```python
from build123d import *

# Parameters (mm, degrees)
F0_R     = 36.4281701053
F0_R_2   = 16.7456603081
F1_DEPTH = 984.504
F2_DEPTH = 127


# Not quite as in the source:
# - a feature of the source that left no trace in its solid (it failed there, or was rolled back) is left out
# - the program builds the solid bodies; features that only make, move or delete a surface that nothing else refers to are left out


with BuildPart() as f1:
    # F0 (on Front) → F1 (new body)
    with BuildSketch(Plane.XZ):
        Circle(F0_R)
        Circle(F0_R_2, mode=Mode.SUBTRACT)
    extrude(amount=F1_DEPTH)

    # F0 (on Front) → F2 (join)
    with BuildSketch(Plane.XZ):
        Polygon((0.0695483181, -76.0122935755), (65.8633513954, -37.9459161775), (65.7938030773, 38.0663773981), (-0.0695483181, 76.0122935755), (-65.8633513954, 37.9459161775), (-65.7938030773, -38.0663773981), align=None)
        Circle(F0_R, mode=Mode.SUBTRACT)
    extrude(amount=F2_DEPTH)


solid = f1.part
```
Work out the finished part from the listing and answer in its coordinate system (mm). A direction names the side the tool comes from. Give positions to 0.01 mm unless a question says otherwise; leave off trailing zeros. Order: outer loops, then holes, each group sorted by start corner. A loop starts at its lowest first (then second) coordinate and runs counter-clockwise, first axis right, second up. Notation, with made-up numbers: (87.25, 19) - (120.25, 19) arc R22 ccw to (120.25, 45) - close; hole circle Ø9 at (26.5, -20). An arc over 180 degrees is marked (long way). One line per item, written item: value. Start each with the question number.
1. For a pull along Z with two mould halves and no side action, classify faces 1 (the face through (-16, -127, 35)), 2 (the face through (-33.323, -62.611, -56.774)), 3 (the face through (-32.506, -62.611, 57.246)), 4 (the face through (-3.63, -485.36, -16.347)) as released by +Z, released by -Z, zero draft, split by the parting line, or undercut.
2. Each of these flat-tipped pins is pushed along its axis until it touches: pin 1 Ø1.5 at (x, z) = (48, 9) entering from -Y; pin 2 Ø5 at (x, y) = (28, -406.5) entering from +Z; pin 3 Ø5 at (x, y) = (10, -725.5) entering from +Z. Where does it stop, or does it pass through?
3. Which of the six approach directions +Z, -Z, +X, -X, +Y, -Y give full straight-line access (tool end or side, diameter ignored) to faces 5 (the face through (34.746, -549.749, 10.942)), 6 (the face through (32.506, -62.611, -57.246))?
4. Section A-A, the plane z = 0 is taken. Write down the section's boundary in (x, y).
5. Consider line 1 (Z direction, x = 0, y = -607); line 2 (Y direction, x = 2, z = 58); line 3 (Z direction, x = -12, y = -146). Determine where each line is inside the solid, lowest interval first.
6. Section C-C, the plane z = -64 is taken. Write down the section's boundary in (x, y).
7. Section B-B, the plane y = -498 is taken. Write down the section's boundary in (x, z), then the cut area to 3 significant figures.
Filled sheet:
1. face 1: zero draft
1. face 2: released by -Z
1. face 3: released by +Z
1. face 4: undercut
2. pin 1: y = -127
2. pin 2: z = 26.01
2. pin 3: z = 35.65
3. face 5: -Y
3. face 6: -Z, +X, +Y, -Y
4. outline: (-65.83, -127) - (-36.43, -127) - (-36.43, -984.5) - (-16.75, -984.5) - (-16.75, 0) - (-65.83, 0) - close; (16.75, -984.5) - (36.43, -984.5) - (36.43, -127) - (65.83, -127) - (65.83, 0) - (16.75, 0) - close
5. line 1: -36.43 to -16.75, 16.75 to 36.43
5. line 2: -127 to 0
5. line 3: -34.39 to -11.68, 11.68 to 34.39
6. outline: (-20.78, -127) - (20.83, -127) - (20.83, 0) - (-20.78, 0) - close
7. outline: circle Ø72.86 at (0, 0); hole circle Ø33.49 at (0, 0)
7. area: 3,290 mm²
